```python
from build123d import *

# Parameters (mm, degrees)
BOSS_EXTRUDE1_DEPTH = 25.4
SHELL1_T            = -3.175


with BuildPart() as part:
    # Sketch1 → Boss-Extrude1 (new body)
    with BuildSketch(Plane(origin=(0, 0, 0), x_dir=(1, 0, 0), z_dir=(0, 1, 0))):
        with BuildLine():
            Line((0, 0), (330.2, 0))
            Line((330.2, 0), (330.2, 76.2))
            ThreePointArc((330.2, 76.2), (318.289658396, 120.65), (285.75, 153.189658396))
            ThreePointArc((285.75, 153.189658396), (165.1, 185.517728463), (44.45, 153.189658396))
            ThreePointArc((44.45, 153.189658396), (11.910341604, 120.65), (0, 76.2))
            Line((0, 76.2), (0, 0))
        make_face()
    extrude(amount=BOSS_EXTRUDE1_DEPTH)

    # Shell1
    shell1_openings = [part.faces().sort_by_distance(p)[0] for p in [
        (165.1, 25.4, -83.209110685),
    ]]
    offset(amount=SHELL1_T, openings=shell1_openings, kind=Kind.INTERSECTION)


solid = part.part
```
Could you check a few things on this model? Use its own coordinates, in mm. A direction names the side the tool comes from. Round coordinates to 2 decimals unless told otherwise and drop trailing zeros. Loops run counter-clockwise (first coordinate to the right, second up) from the corner with the lowest first, then second, coordinate; pieces in that order, holes last. Notation, with made-up numbers: M -15.5,68.25 L 0.5,68.25 A15 ccw 0.5,82.25 Z; hole C 74.25,65 d9. An arc over 180 degrees is marked long. Write item = value, one per line.
1. Which directions (+Z, -Z, +X, -X, +Y, -Y) give clear straight access to the entire face, cutting with the end or side of a thin tool? Please do faces 1 (the face through (14.98, 14.13, -119.61)), 2 (the face through (163, 0, -94)).
Results below:
face_1 = +Y
face_2 = +Z, -Z, +X, -X, -Y
2. I need wall thicknesses on probe 1 along X at (y, z) = (12, -46.5) (3 decimals); probe 2 along Y at (x, z) = (240.5, -167.5) (3 decimals); probe 3 along Z at (x, y) = (73.5, 5) (3 decimals). Which ranges of each line are inside material? Lowest first, please.
Results below:
probe_1 = 0 to 3.175, 327.025 to 330.2
probe_2 = 0 to 3.175
probe_3 = -167.456 to -164.02, -3.175 to 0
3. Thinking about a two-plate mould opening in X: for faces 3 (the face through (163, 13, 0)), 4 (the face through (166.846, 14.132, -182.336)), 5 (the face through (163, 3.175, -94)), 6 (the face through (0, 13, -39)), which applies, +X half, -X half, draft (parallel to the pull), parting line (faces both ways), or undercut?
Results below:
face_3 = draft
face_4 = undercut
face_5 = undercut
face_6 = -X half
4. I want a section at B-B, the plane z = -16.5. Write out the boundary of the cut face in (x, y) (3 decimals), and give its area (3 significant figures).
Results below:
outline = M 0,0 L 330.2,0 L 330.2,25.4 L 327.025,25.4 L 327.025,3.175 L 3.175,3.175 L 3.175,25.4 L 0,25.4 Z
area = 1,190 mm²
5. I want a section at C-C, the plane x = 103.5. Write out the boundary of the cut face in (y, z) (3 decimals), and give its area (3 significant figures).
Results below:
outline = M 0,-177.523 L 25.4,-177.523 L 25.4,-174.237 L 3.175,-174.237 L 3.175,-3.175 L 25.4,-3.175 L 25.4,0 L 0,0 Z
area = 707 mm²
6. Will these pins go through, and if not, where does the flat tip stop? P1, Ø2, axis at y = 20.5, z = -95, coming from the -X side; P2, Ø1, axis at x = 255, z = -83.5, coming from the +Y side (3 decimals); P3, Ø2, axis at x = 65.5, z = -147, coming from the -Y side; P4, Ø1.5, axis at x = 207, y = 11, coming from the -Z side.
Results below:
P1 = 1.8
P2 = 3.175
P3 = 0
P4 = -181.98
